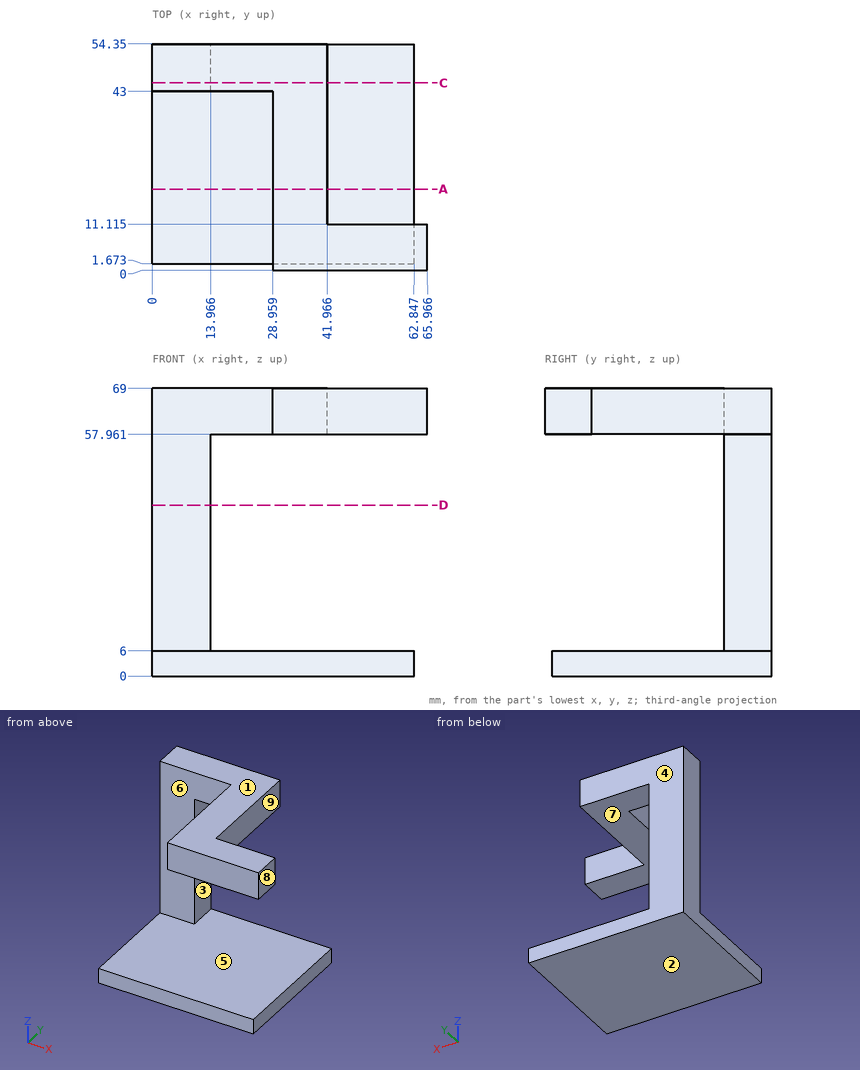
Geometry check sheet. Reference: drawing and pictorial views, mm from the part's lowest x, y, z. A direction names the side the tool comes from. Give positions to 0.01 mm unless a question says otherwise; leave off trailing zeros. Loops run counter-clockwise (first coordinate to the right, second up) from the corner with the lowest first, then second, coordinate; pieces in that order, holes last. Notation, with made-up numbers: (45, 68.5) -> (82, 68.5) arc R21 cw to (82, 77.5) -> close; hole circle Ø1 at (70, -8.5). An arc over 180 degrees is marked (long way). Answer in a Markdown table with one row per item. Add a question column.
1) Cross-section at A-A on y = 19.5. Record the boundary of the cut face in (x, z), and give its area (3 significant figures).
2) Draft check along Z on the marked faces 1, 2, 3 and 4. Enter one of: pulls with the +Z half, pulls with the -Z half, needs draft (parallel to the pull), parting line crosses it, or undercut.
3) Cross-section at D-D on z = 41. Record the boundary of the cut face in (x, y).
4) Material ranges on probe 1 along Z at (x, y) = (51, 7); probe 2 along X at (y, z) = (48, 4); probe 3 along Y at (x, z) = (3.5, 14), recorded low to high. Write a range as from..to.
5) Gauge pin test, flat ends, axial feed: P1, Ø3.5, axis at y = 18.5, z = 66, coming from the -X side; P2, Ø3.5, axis at y = 28.5, z = 61.5, coming from the +X side; P3, Ø3.5, axis at x = 50, z = 63, coming from the +Y side (3 decimals). Record the tip position at first contact, or that the pin passes through.
6) Set-up check for the marked faces 5, 6, 7, 8 and 9: record each of +Z, -Z, +X, -X, +Y, -Y from which the full face is reachable in a straight line by a thin tool's end or side.
7) Cross-section at C-C on y = 45. Record the boundary of the cut face in (x, z), and give its area (3 significant figures).
Outcome:
| question | item | result |
|---|---|---|
| 1 | outline | (0, 0) -> (62.85, 0) -> (62.85, 6) -> (0, 6) -> close; (28.96, 57.96) -> (41.97, 57.96) -> (41.97, 69) -> (28.96, 69) -> close |
| 1 | area | 521 mm^2 |
| 2 | face 1 | pulls with the +Z half |
| 2 | face 2 | pulls with the -Z half |
| 2 | face 3 | undercut |
| 2 | face 4 | needs draft |
| 3 | outline | (0, 43) -> (13.97, 43) -> (13.97, 54.35) -> (0, 54.35) -> close |
| 4 | probe 1 | z = 0..6, 57.96..69 |
| 4 | probe 2 | x = 0..62.85 |
| 4 | probe 3 | y = 43..54.35 |
| 5 | P1 | stops at x = 28.96 |
| 5 | P2 | stops at x = 41.97 |
| 5 | P3 | stops at y = 11.115 |
| 6 | face 5 | +X, -Y |
| 6 | face 6 | +Z, -X, -Y |
| 6 | face 7 | +X, +Y, -Y |
| 6 | face 8 | +Z, -Z, +X, +Y, -Y |
| 6 | face 9 | +Z, +X, +Y |
| 7 | outline | (0, 0) -> (62.85, 0) -> (62.85, 6) -> (13.97, 6) -> (13.97, 57.96) -> (41.97, 57.96) -> (41.97, 69) -> (0, 69) -> close |
| 7 | area | 1,570 mm^2 |
